Verification items for the finished model (mm, model axes). Face numbers are marked on the shaded views. A direction names the side the tool comes from. Give positions to 0.01 mm unless a question says otherwise; leave off trailing zeros. Write each loop counter-clockwise with the first axis right and the second up, starting at its lowest first coordinate (ties: lowest second). Pieces come first, ordered by that corner, then holes. Notation, with made-up numbers: (75.25, -35) - (102.25, -35) arc R14 ccw to (102.25, -23) - close; hole circle Ø9 at (43.5, -24.75). An arc over 180 degrees is marked (long way). Put each result on its own line as item: value.
from build123d import *

# Parameters (mm, degrees)
SKETCH_W        = 94
SKETCH_H        = 20
EXTRUDE_DEPTH   = 3
SKETCH001_R     = 1.25
HOLE_DEPTH      = 3
FILLET_R        = 6
SKETCH002_W     = 23.4
SKETCH002_H     = 21
POCKET_DEPTH    = 1.5
SKETCH003_W     = 23.4
SKETCH003_H     = 21
POCKET001_DEPTH = 1.5


with BuildPart() as part:
    # Sketch → Extrude (new body)
    with BuildSketch(Plane.XY):
        with Locations((0.620003, 10.899999)):
            Rectangle(SKETCH_W, SKETCH_H)
    extrude(amount=EXTRUDE_DEPTH)

    # Sketch001 (on Face6 of BaseFeature) → Hole (cut)
    with BuildSketch(Plane.XY.offset(3)):
        with Locations((-38.549999, 10.83)):
            Circle(SKETCH001_R)
        with Locations((39.800001, 10.823599)):
            Circle(SKETCH001_R)
    extrude(amount=-HOLE_DEPTH, mode=Mode.SUBTRACT)

    # Fillet
    fillet_edges = [part.edges().sort_by_distance(p)[0] for p in [
        (-46.379997, 0.899999, 1.5),
        (-46.379997, 20.899999, 1.5),
        (47.620003, 20.899999, 1.5),
        (47.620003, 0.899999, 1.5),
    ]]
    fillet(fillet_edges, radius=FILLET_R)

    # Sketch002 (on Face5 of Fillet) → Pocket (cut)
    with BuildSketch(Plane.XY.offset(3)):
        with Locations((-34.701599, 10.700001)):
            Rectangle(SKETCH002_W, SKETCH002_H)
    extrude(amount=-POCKET_DEPTH, mode=Mode.SUBTRACT)

    # Sketch003 (on Face4 of Pocket) → Pocket001 (cut)
    with BuildSketch(Plane.XY.offset(3)):
        with Locations((36.4, 10.699637)):
            Rectangle(SKETCH003_W, SKETCH003_H)
    extrude(amount=-POCKET001_DEPTH, mode=Mode.SUBTRACT)


solid = part.part
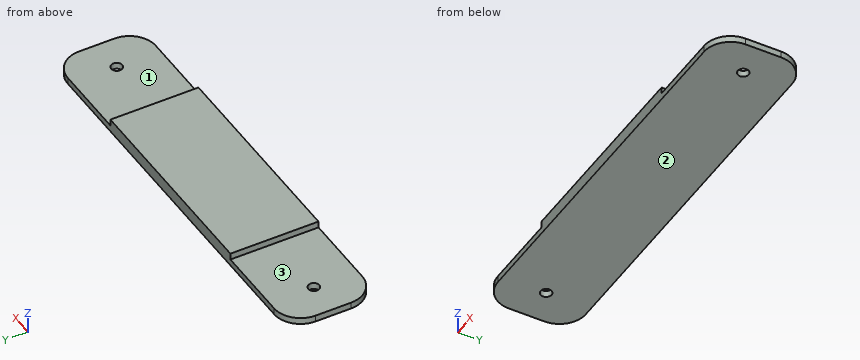
Q1. Section check C-C, the plane y = 13.25. Record the cut outline in (x, z).
Answers follow:
outline: (-46.38, 0) - (47.62, 0) - (47.62, 1.5) - (24.7, 1.5) - (24.7, 3) - (-23, 3) - (-23, 1.5) - (-46.38, 1.5) - close
Q2. Section check B-B, the plane z = 0.55. Record the cut outline in (x, y).
Answers follow:
outline: (-46.38, 6.9) arc R6 ccw to (-40.38, 0.9) - (41.62, 0.9) arc R6 ccw to (47.62, 6.9) - (47.62, 14.9) arc R6 ccw to (41.62, 20.9) - (-40.38, 20.9) arc R6 ccw to (-46.38, 14.9) - close; hole circle Ø2.5 at (-38.55, 10.83); hole circle Ø2.5 at (39.8, 10.82)
Q3. Section check D-D, the plane y = 17.5. Record the cut outline in (x, z).
Answers follow:
outline: (-45.79, 0) - (47.03, 0) - (47.03, 1.5) - (24.7, 1.5) - (24.7, 3) - (-23, 3) - (-23, 1.5) - (-45.79, 1.5) - close
Q4. Go/stop test with flat-tipped pins: pin 1 Ø1.5 at (y, z) = (18, 1) entering from -X; pin 2 Ø3 at (x, y) = (39.8, 10.82) entering from +Z. Record where each tip stops, or that it passes through.
Answers follow:
pin 1: stops at x = -45.9
pin 2: stops at z = 1.5
Q5. Scan lines: line 1 along Y through (x, z) = (-38.55, 1.05); line 2 along Z through (x, y) = (40.5, 18.25); line 3 along X through (y, z) = (10.25, 1.15). Record each from-to range of solid material in increasing order.
Answers follow:
line 1: y = 0.9 to 9.58, 12.08 to 20.9
line 2: z = 0 to 1.5
line 3: x = -46.38 to -39.66, -37.44 to 38.69, 40.91 to 47.62
Q6. Set-up check for the marked faces 1, 2 and 3: record each of +Z, -Z, +X, -X, +Y, -Y from which the full face is reachable in a straight line by a thin tool's end or side.
Answers follow:
face 1: +Z, +X, +Y, -Y
face 2: -Z, +X, -X, +Y, -Y
face 3: +Z, -X, +Y, -Y
Q7. Section check A-A, the plane x = -38.55. Record the cut outline in (y, z).
Answers follow:
outline: (0.9, 0) - (9.58, 0) - (9.58, 1.5) - (0.9, 1.5) - close; (12.08, 0) - (20.9, 0) - (20.9, 1.5) - (12.08, 1.5) - close
